Could you check a few things on this model? Use its own coordinates, in mm. A direction names the side the tool comes from. Give positions to 0.01 mm unless a question says otherwise; leave off trailing zeros. Loops run counter-clockwise (first coordinate to the right, second up) from the corner with the lowest first, then second, coordinate; pieces in that order, holes last. Notation, with made-up numbers: M 10,42 L 45,42 A6 cw 45,51 Z; hole C -16.5,-10.5 d4. An arc over 180 degrees is marked long. Answer in a Markdown table with one row per item. Add a question column.
```python
from build123d import *

# Parameters (mm, degrees)
BOSS_EXTRUDE1_DEPTH = 25.4
SKETCH3_R           = 63.5
BOSS_EXTRUDE2_DEPTH = 127
BOSS_EXTRUDE3_DEPTH = 50.8
SKETCH5_R           = 101.6
BOSS_EXTRUDE4_DEPTH = 25.4
SKETCH6_R           = 63.5
BOSS_EXTRUDE5_DEPTH = 101.6


with BuildPart() as part:
    # Sketch2 → Boss-Extrude1 (new body)
    with BuildSketch(Plane.XY):
        with BuildLine():
            Line((0, 63.5), (-459.135608438, 63.5))
            ThreePointArc((-459.135608438, 63.5), (-522.635608438, 0), (-459.135608438, -63.5))
            Line((-459.135608438, -63.5), (0, -63.5))
            ThreePointArc((0, -63.5), (63.5, 0), (0, 63.5))
        make_face()
    extrude(amount=BOSS_EXTRUDE1_DEPTH)

    # Sketch3 → Boss-Extrude2 (add)
    with BuildSketch(Plane.XY.offset(25.4)):
        with Locations(Location((0, 0, 0), (0, 0, 90))):
            Circle(SKETCH3_R)
    extrude(amount=BOSS_EXTRUDE2_DEPTH)

    # Sketch4 → Boss-Extrude3 (add)
    with BuildSketch(Plane.XY.offset(152.4)):
        with BuildLine():
            Line((-51.372579143, 37.324363521), (-156.920582469, -107.95))
            ThreePointArc((-156.920582469, -107.95), (0, -190.439904187), (156.920582469, -107.95))
            Line((156.920582469, -107.95), (51.372579143, 37.324363521))
            ThreePointArc((51.372579143, 37.324363521), (0, 63.5), (-51.372579143, 37.324363521))
        make_face()
    extrude(amount=BOSS_EXTRUDE3_DEPTH)

    # Sketch5 → Boss-Extrude4 (add)
    with BuildSketch(Plane.XY.offset(203.2)):
        with Locations(Location((0, 19.05, 0), (0, 0, 203.016562949))):
            Circle(SKETCH5_R)
    extrude(amount=BOSS_EXTRUDE4_DEPTH)

    # Sketch6 → Boss-Extrude5 (add)
    with BuildSketch(Plane.XY.offset(228.6)):
        with Locations(Location((0, 0, 0), (0, 0, 144))):
            Circle(SKETCH6_R)
    extrude(amount=BOSS_EXTRUDE5_DEPTH)


solid = part.part
```
Item 1: Suppose I cut it at B-B (z = 189). List the corners of the cut face in (x, y) for me, then the cut area to 3 significant figures.
Item 2: Suppose I cut it at C-C (x = -36). List the corners of the cut face in (y, z) for me, then the cut area to 3 significant figures.
Item 3: Suppose I cut it at D-D (y = 93). List the corners of the cut face in (x, z) for me, then the cut area to 3 significant figures.
Item 4: I need wall thicknesses on L1, parallel to Z at x = -145.5, y = -50.5; L2, parallel to Z at x = -68, y = 15; L3, parallel to Y at x = -99, z = 14.5. Which ranges of each line are inside material? Lowest first, please.
Item 5: For P1, Ø8, axis at x = -28.5, z = 257.5, coming from the -Y side; P2, Ø12, axis at y = -30, z = 156.5, coming from the +X side; P3, Ø3, axis at x = 58, z = 101, coming from the -Y side, each with a flat end and sliding along its axis, tell me the tip position at first contact or that it passes through.
Item 6: If we mould it in two halves opening along Z, with no side actions, what happens to faces 5 (the face through (5, 69, 228.6)), 6 (the face through (2, 76, 203.2)), 7 (the face through (-226, 63.5, 13))? For each: +Z half, -Z half, draft (parallel to the pull), parting line (faces both ways), or undercut.
Item 7: For faces 1 (the face through (12.64, -62.23, 278.69)), 2 (the face through (104.885, -36.33, 177.444)), 3 (the face through (-233, -63.5, 13)), 4 (the face through (-103.41, -34.3, 177.44)), which set-ups out of +Z, -Z, +X, -X, +Y, -Y let a thin tool reach every point of the face, with its end or its side?
Item 8: Suppose I cut it at A-A (x = -127.5). List the corners of the cut face in (y, z) for me.
Values found:
| question | item | result |
|---|---|---|
| 1 | outline | M -156.92,-107.95 A190.5 ccw 156.92,-107.95 L 51.37,37.32 A63.5 ccw -51.37,37.32 Z |
| 1 | area | 50,300 mm² |
| 2 | outline | M -187.01,152.4 L -52.31,152.4 L -52.31,25.4 L -63.5,25.4 L -63.5,0 L 63.5,0 L 63.5,25.4 L 52.31,25.4 L 52.31,203.2 L 114.06,203.2 L 114.06,228.6 L 52.31,228.6 L 52.31,330.2 L -52.31,330.2 L -52.31,228.6 L -75.96,228.6 L -75.96,203.2 L -187.01,203.2 Z |
| 2 | area | 44,100 mm² |
| 3 | outline | M -69.67,203.2 L 69.67,203.2 L 69.67,228.6 L -69.67,228.6 Z |
| 3 | area | 3,540 mm² |
| 4 | L1 | 0 to 25.4 |
| 4 | L2 | 0 to 25.4, 203.2 to 228.6 |
| 4 | L3 | -63.5 to 63.5 |
| 5 | P1 | y = -58.58 |
| 5 | P2 | x = 104.65 |
| 5 | P3 | y = -28.98 |
| 6 | face 5 | +Z half |
| 6 | face 6 | undercut |
| 6 | face 7 | draft |
| 7 | face 1 | +Z |
| 7 | face 2 | -Z, +X, +Y |
| 7 | face 3 | -Z, +X, -X, -Y |
| 7 | face 4 | -X, +Y |
| 8 | outline | M -141.48,152.4 L -67.46,152.4 L -67.46,203.2 L -141.48,203.2 Z; M -63.5,0 L 63.5,0 L 63.5,25.4 L -63.5,25.4 Z |
